from build123d import *

# Parameters (mm, degrees)
F0_W      = 18.923
F0_H      = 19.05
F0_W_2    = 4.5085
F1_DEPTH  = 6.35
F3_DEPTH  = 25.4
F4_W      = 9.652
F4_H      = 19.05
F5_DEPTH  = 32.385
F7_DEPTH  = 25.4
F8_R      = 3.4036
F9_DEPTH  = 6.35
F11_DEPTH = 25.4


with BuildPart() as f1:
    # F0 (on Top) → F1 (new body)
    with BuildSketch(Plane.XY):
        with Locations((9.4615, 9.525)):
            Rectangle(F0_W, F0_H)
        with Locations((-2.25425, 9.525)):
            Rectangle(F0_W_2, F0_H)
        with Locations((21.17725, 9.525)):
            Rectangle(F0_W_2, F0_H)
    extrude(amount=-F1_DEPTH)

    # F2 (on face) → F3 (join)
    with BuildSketch(Plane.XY):
        Polygon((-2.5273, 10.287), (0, 10.287), (0, 15.7734), (-2.426286, 15.7734), (-2.426286, 14.4272), (-4.5085, 14.4272), (-4.5085, 11.6332), (-2.5273, 11.6332), align=None)
        Polygon((21.4503, 7.4168), (21.4503, 8.763), (18.923, 8.763), (18.923, 3.2766), (21.524463, 3.2766), (21.524463, 4.6228), (23.4315, 4.6228), (23.4315, 7.4168), align=None)
        Polygon((18.923, 15.7734), (18.923, 10.287), (21.4503, 10.287), (21.4503, 11.6332), (23.4315, 11.6332), (23.4315, 14.4272), (21.349286, 14.4272), (21.349286, 15.7734), align=None)
        Polygon((0, 3.2766), (0, 8.763), (-2.5273, 8.763), (-2.5273, 7.4168), (-4.5085, 7.4168), (-4.5085, 4.6228), (-2.601463, 4.6228), (-2.601463, 3.2766), align=None)
    extrude(amount=F3_DEPTH)

    # F4 (on face) → F5 (join)
    with BuildSketch(Plane(origin=(0, 0, -6.35), x_dir=(1, 0, 0), z_dir=(0, 0, -1))):
        with Locations((9.4615, -9.525)):
            Rectangle(F4_W, F4_H)
    extrude(amount=F5_DEPTH)

    # F6 (on face) → F7 (cut)
    with BuildSketch(Plane(origin=(4.6355, 0, 0), x_dir=(0, -1, 0), z_dir=(-1, 0, 0))):
        Polygon((-19.05, -38.735), (-3.4036, -38.735), (-19.05, -10.795), align=None)
    extrude(amount=-F7_DEPTH, mode=Mode.SUBTRACT)

    # F8 (on face) → F9 (cut)
    with BuildSketch(Plane(origin=(0, 19.104141, -10.698319), x_dir=(-1, 0, 0), z_dir=(0, 0.872506, -0.488603))):
        with Locations((-9.638287, -11.434614)):
            Circle(F8_R)
    extrude(amount=-F9_DEPTH, mode=Mode.SUBTRACT)

    # F10 (on face) → F11 (cut)
    with BuildSketch(Plane(origin=(4.6355, 0, 0), x_dir=(0, -1, 0), z_dir=(-1, 0, 0))):
        Polygon((-7.264855, -11.930685), (-10.212355, -13.581285), (-5.819029, -21.42651), (-2.871529, -19.77591), align=None)
    extrude(amount=-F11_DEPTH, mode=Mode.SUBTRACT)


solid = f1.part
Build history of the part. All positions in model axes, mm. A direction names the side the tool comes from. Coordinates: 2 decimals unless noted, no trailing zeros. Order: outer loops, then holes, each group sorted by start corner. A loop starts at its lowest first (then second) coordinate and runs counter-clockwise, first axis right, second up. Notation, with made-up numbers: (-27.75, -28) -> (-11.75, -28) arc R16 ccw to (-11.75, -18) -> close; hole circle Ø7 at (62.5, -34.75). An arc over 180 degrees is marked (long way). One line per item, written item: value.
(1) Probe line 1 (X direction, y = 7.25, z = 11); line 2 (X direction, y = 8, z = 10.5); line 3 (X direction, y = 13.75, z = -6.5). List the from-to ranges inside material, lowest first. Write a range as [from, to].
Checked values:
line 1: [-4.51, 0], [18.92, 23.43]
line 2: [-2.53, 0], [18.92, 21.45]
line 3: [4.64, 14.29]
(2) Slice it at D-D, the plane x = 8.75. List the corners of the cut face in (y, z) (3 decimals), plus the area to 3 significant figures.
Checked values:
outline: (0, -38.735) -> (3.404, -38.735) -> (11.912, -23.542) -> (6.372, -20.439) -> (5.819, -21.427) -> (2.872, -19.776) -> (7.265, -11.931) -> (10.212, -13.581) -> (9.583, -14.706) -> (15.123, -17.808) -> (19.05, -10.795) -> (19.05, 0) -> (0, 0) -> close
area: 447 mm2
(3) Mould opens along X. For faces 1 (the flat face through (4.635, 8, -19)), 2 (the flat face through (-1, 8.763, 13)), 3 (the flat face through (9, 10, 0)), 4 (the flat face through (0, 6, 13)) say: pulls with the +X half, pulls with the -X half, needs draft (parallel to the pull), parting line crosses it, or undercut.
Checked values:
face 1: pulls with the -X half
face 2: needs draft
face 3: undercut
face 4: undercut
(4) Slice it at C-C, the plane z = -13. List the corners of the cut face in (x, y), plus the area to 3 significant figures.
Checked values:
outline: (4.64, 0) -> (14.29, 0) -> (14.29, 6.67) -> (4.64, 6.67) -> close; (4.64, 9.17) -> (14.29, 9.17) -> (14.29, 17.82) -> (4.64, 17.82) -> close
area: 148 mm2
(5) Tool access for faces 5 (the flat face through (9.394, 8.718, -12.744)), 6 (the flat face through (-2.426, 15, 13)), 7 (the flat face through (21.524, 4, 13)): list every direction of +Z, -Z, +X, -X, +Y, -Y with a clear straight run to the whole face (end or side of a thin tool).
Checked values:
face 5: +X, -X
face 6: +Z, -X, +Y
face 7: +Z, +X, -Y
(6) Drop flat-ended pins along their axis: pin 1 Ø4 at (x, y) = (10, 7) entering from +Z; pin 2 Ø7.5 at (x, y) = (0, 13) entering from -Z; pin 3 Ø2 at (x, z) = (-0.5, 7.5) entering from -Y; pin 4 Ø6 at (x, z) = (12.5, 4) entering from +Y. Give the stop position or say it passes through.
Checked values:
pin 1: z = 0
pin 2: z = -6.35
pin 3: y = 3.28
pin 4: through
(7) Slice it at B-B, the plane x = -1.25. List the corners of the cut face in (y, z), plus the area to 3 significant figures.
Checked values:
outline: (0, -6.35) -> (19.05, -6.35) -> (19.05, 0) -> (15.77, 0) -> (15.77, 25.4) -> (10.29, 25.4) -> (10.29, 0) -> (8.76, 0) -> (8.76, 25.4) -> (3.28, 25.4) -> (3.28, 0) -> (0, 0) -> close
area: 400 mm2
(8) Slice it at A-A, the plane z = 6. Count the separate pieces of the cut face and the enclosed holes in it, plus the area to 3 significant figures.
Checked values:
separate pieces: 4
enclosed holes: 0
area: 77.5 mm2
